Read the model definition and answer for the solid it produces. Units are mm, in the model's axes. Face numbers are marked on the shaded views. A direction names the side the tool comes from. Coordinates: 2 decimals unless noted, no trailing zeros. Order: outer loops, then holes, each group sorted by start corner. A loop starts at its lowest first (then second) coordinate and runs counter-clockwise, first axis right, second up. Notation, with made-up numbers: (69, -19.5) - (76, -19.5) arc R19 ccw to (76, -4.5) - close; hole circle Ø1 at (-19, 20.5). An arc over 180 degrees is marked (long way). Use one line per item in the form item = value.
```python
from build123d import *

# Parameters (mm, degrees)
IZIM3_W               = 6
IZIM3_H               = 3
IZIM4_W               = 20
IZIM4_H               = 5
KES_EKSTR_ZYON1_DEPTH = 3


with BuildPart() as part:
    # Çizim2 → Döndür1 (revolve)
    with BuildSketch(Plane.XY, mode=Mode.PRIVATE) as d_nd_r1_sk:
        Polygon((0, 0), (0, 10), (-100, 10), (-100, 12.5), (-110, 12.5), (-110, 9.5), (-130, 9.5), (-130, 0), align=None)
    revolve(d_nd_r1_sk.sketch.rotate(Axis((-130, 0, 0), (1, 0, 0)), 90), axis=Axis((-130, 0, 0), (1, 0, 0)))

    # Çizim3 → Kes-Döndür1 (revolve, cut)
    with BuildSketch(Plane.XY, mode=Mode.PRIVATE) as kes_d_nd_r1_sk:
        with Locations((-120, 8)):
            Rectangle(IZIM3_W, IZIM3_H)
    revolve(kes_d_nd_r1_sk.sketch.rotate(Axis((-130, 0, 0), (1, 0, 0)), 90), axis=Axis((-130, 0, 0), (1, 0, 0)), mode=Mode.SUBTRACT)

    # Çizim4 → Kes-Ekstrüzyon1 (cut, symmetric)
    with BuildSketch(Plane.XY):
        with Locations((-10, 9.5)):
            Rectangle(IZIM4_W, IZIM4_H)
    extrude(amount=KES_EKSTR_ZYON1_DEPTH, both=True, mode=Mode.SUBTRACT)


solid = part.part
```
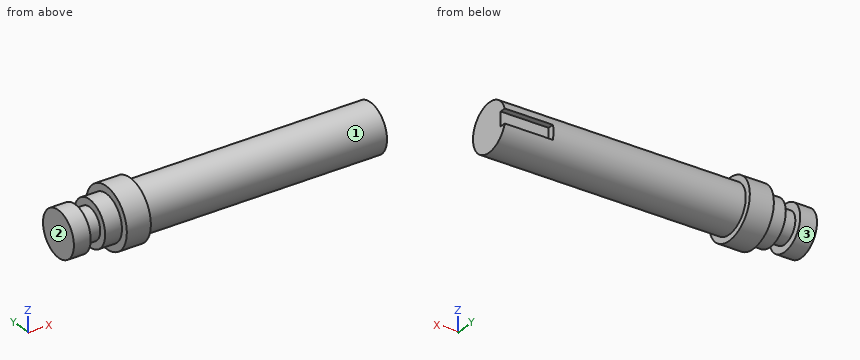
(1) Which of the six approach directions +Z, -Z, +X, -X, +Y, -Y give full straight-line access (tool end or side, diameter ignored) to the marked faces 1, 2 and 3?
Answer list:
face_1 = +X
face_2 = +Z, -Z, -X, +Y, -Y
face_3 = -X
(2) Section D-D, the plane z = 5.25 is taken. Write down the section's boundary in (x, y).
Answer list:
outline = (-130, -7.92) - (-123, -7.92) - (-123, -3.83) - (-117, -3.83) - (-117, -7.92) - (-110, -7.92) - (-110, -11.34) - (-100, -11.34) - (-100, -8.51) - (0, -8.51) - (0, 8.51) - (-100, 8.51) - (-100, 11.34) - (-110, 11.34) - (-110, 7.92) - (-117, 7.92) - (-117, 3.83) - (-123, 3.83) - (-123, 7.92) - (-130, 7.92) - close
(3) Straight lines are drawn through the part: L1, parallel to X at y = -5.5, z = -3.75; L2, parallel to X at y = 9, z = -7; L3, parallel to Y at x = -124.5, z = 2.25. For each, find the intervals that lie inside material, in ascending order.
Answer list:
L1 = -130 to -123, -117 to 0
L2 = -110 to -100
L3 = -9.23 to 9.23
(4) Section B-B, the plane z = 0 is taken. Write down the section's boundary in (x, y).
Answer list:
outline = (-130, -9.5) - (-123, -9.5) - (-123, -6.5) - (-117, -6.5) - (-117, -9.5) - (-110, -9.5) - (-110, -12.5) - (-100, -12.5) - (-100, -10) - (0, -10) - (0, 7) - (-20, 7) - (-20, 10) - (-100, 10) - (-100, 12.5) - (-110, 12.5) - (-110, 9.5) - (-117, 9.5) - (-117, 6.5) - (-123, 6.5) - (-123, 9.5) - (-130, 9.5) - close
(5) Section C-C, the plane x = -51 is taken. Write down the section's boundary in (y, z), then the cut area to 3 significant figures.
Answer list:
outline = circle Ø20 at (0, 0)
area = 314 mm2
(6) Given pin 1 Ø2 at (x, y) = (-81, 0.5) entering from -Z; pin 2 Ø2 at (x, z) = (-104, 1) entering from +Y; pin 3 Ø1.5 at (x, y) = (-51.5, -6.5) entering from -Z; pin 4 Ø4 at (x, z) = (-79, -8.5) entering from -Y, each flat-ended and moving along its own axis, determine where each tip first touches the part or whether it passes through.
Answer list:
pin_1 = -10
pin_2 = 12.5
pin_3 = -8.18
pin_4 = -7.6
(7) Section A-A, the plane y = 0 is taken. Write down the section's boundary in (x, z), then the cut area to 3 significant figures.
Answer list:
outline = (-130, -9.5) - (-123, -9.5) - (-123, -6.5) - (-117, -6.5) - (-117, -9.5) - (-110, -9.5) - (-110, -12.5) - (-100, -12.5) - (-100, -10) - (0, -10) - (0, 10) - (-100, 10) - (-100, 12.5) - (-110, 12.5) - (-110, 9.5) - (-117, 9.5) - (-117, 6.5) - (-123, 6.5) - (-123, 9.5) - (-130, 9.5) - close
area = 2,590 mm2
